from build123d import *

# Parameters (mm, degrees)
F0_W     = 71.4285714286
F0_H     = 3.175
F1_DEPTH = 3.175


# Not quite as in the source:
# - ends of sketch curves that miss each other by under 0.0002 mm in the source are joined


with BuildPart() as f1:
    # F0 (on Front) → F1 (new body)
    with BuildSketch(Plane.XZ):
        Polygon((-260, 10), (-260, -10), (160, -10), (160, 10), (-81.8902254105, 10), (-91.575, 10), (-190, 10), (-197.4899102798, 10), align=None)
        with Locations((-214.2857571429, 0)):
            Rectangle(F0_W, F0_H, mode=Mode.SUBTRACT)
        Polygon((-35.7142857143, 1.5875), (-35.7142857143, -1.5875), (-107.1428714286, -1.5875), (-107.1428857143, 1.5875), align=None, mode=Mode.SUBTRACT)
        with Locations((71.4285857143, 0)):
            Rectangle(F0_W, F0_H, mode=Mode.SUBTRACT)
        Polygon((-190, 25), (-197.4899102798, 10), (-190, 10), (-190, 21.825), align=None)
        Polygon((-190, 21.825), (-190, 10), (-91.575, 10), (-91.575, 21.825), (-111.26, 21.825), (-111.26, 25), (-130.945, 25), (-130.945, 21.825), (-150.63, 21.825), (-150.63, 25), (-170.315, 25), (-170.315, 21.825), align=None)
        Polygon((-91.575, 10), (-81.8902254105, 10), (-91.575, 25), (-91.575, 21.825), align=None)
    extrude(amount=F1_DEPTH)


solid = f1.part
CAD build for the part. Positions are in the model's coordinates, mm. Round coordinates to 2 decimals unless told otherwise and drop trailing zeros. Write each loop counter-clockwise with the first axis right and the second up, starting at its lowest first coordinate (ties: lowest second). Pieces come first, ordered by that corner, then holes.
(1) Slice it at A-A, the plane x = 71. Write the cut outline in (y, z) (1 decimal).
(2) Drop flat-ended pins along their axis: P1, Ø1, axis at x = -214.5, y = -1, coming from the +Z side; P2, Ø1.6, axis at y = -2, z = 24, coming from the +X side; P3, Ø4, axis at x = 6, z = 3.5, coming from the +Y side; P4, Ø1, axis at y = -2.5, z = 21.5, coming from the -X side. Give the stop position or say it passes through.
(3) Slice it at B-B, the plane y = -2.35. Count the separate pieces of the cut face and the enclosed holes in it, and give its area (3 significant figures).
(4) Probe line 1 along Z through (x, y) = (85.5, -2.4); line 2 along X through (y, z) = (-2.9, 0); line 3 along Z through (x, y) = (-186.5, -1.9) (1 decimal). List the from-to ranges inside material, lowest first.
(5) Slice it at C-C, the plane x = -13. Write the cut outline in (y, z) (3 decimals), and give its area (3 significant figures).
From the geometry:
1. outline: (-3.2, -10) - (0, -10) - (0, -1.6) - (-3.2, -1.6) - close; (-3.2, 1.6) - (0, 1.6) - (0, 10) - (-3.2, 10) - close
2. P1: stops at z = 10
2. P2: stops at x = -90.41
2. P3: stops at y = 0
2. P4: stops at x = -192
3. separate pieces: 1
3. enclosed holes: 3
3. area: 9,140 mm2
4. line 1: z = -10 to -1.59, 1.59 to 10
4. line 2: x = -260 to -250, -178.57 to -107.14, -35.71 to 35.71, 107.14 to 160
4. line 3: z = -10 to -1.6, 1.6 to 21.8
5. outline: (-3.175, -10) - (0, -10) - (0, 10) - (-3.175, 10) - close
5. area: 63.5 mm2
